Part model, mm, in its own coordinate system. A direction names the side the tool comes from. Give positions to 0.01 mm unless a question says otherwise; leave off trailing zeros. Order: outer loops, then holes, each group sorted by start corner. A loop starts at its lowest first (then second) coordinate and runs counter-clockwise, first axis right, second up. Notation, with made-up numbers: (24, 21.5) -> (35, 21.5) arc R31 ccw to (35, 60.5) -> close; hole circle Ø4 at (70, 53). An arc over 180 degrees is marked (long way). Write item = value, one per line. Start each with the question number.
(1) Probe line 1 along X through (y, z) = (55.5, -45.5); line 2 along X through (y, z) = (41, -36.5); line 3 along X through (y, z) = (91, 16). List the from-to ranges inside material, lowest first. Write a range as from..to.
(2) Flat gauge pins, fed straight in: pin 1 (1 mm diameter, centred on x = 61.5, z = -11.5, fed in from +Y); pin 2 (3 mm diameter, centred on x = 56, z = -33.5, fed in from +Y); pin 3 (1.5 mm diameter, centred on x = 82, y = 50.5, fed in from -Z). Where does each tip first touch, or does it go through?
(3) Saw through at A-A, the plane z = -68. List the corners of the cut face in (x, y), then the cut area to 3 significant figures.
(4) Which spindle directions (+Z, -Z, +X, -X, +Y, -Y) get a long thin tool onto all of the face, cutting with end or side? Do faces 5 (the cylindrical face through (56.1, 69.3, -48.9)), 6 (the flat face through (-9, 101.6, -35)). Say none if no direction does.
(5) Two-plate mould, pull along Y, no slides. Class faces 1 (the flat face through (33.566, 63.554, -20.049)), 2 (the flat face through (96.799, 21, -33)), 3 (the cylindrical face through (-8.706, 99.69, 24.452)), 4 (the cylindrical face through (34.07, 81.99, -33.91)): pulls with the +Y half, pulls with the -Y half, needs draft (parallel to the pull), parting line crosses it, or undercut.
from build123d import *

# Parameters (mm, degrees)
SKETCH1_W           = 120.65
SKETCH1_H           = 120.65
BOSS_EXTRUDE1_DEPTH = 101.6
CUT_EXTRUDE1_DEPTH  = 120.65
CUT_EXTRUDE2_DEPTH  = 31.75
CUT_EXTRUDE3_DEPTH  = 6.35
CUT_EXTRUDE3_TAPER  = 45
FILLET1_R           = 6.35
FILLET2_R           = 2.54


with BuildPart() as part:
    # Sketch1 → Boss-Extrude1 (new body)
    with BuildSketch(Plane(origin=(0, 0, 0), x_dir=(1, 0, 0), z_dir=(0, 1, 0))):
        with Locations((36.473705191, 34.061776503)):
            Rectangle(SKETCH1_W, SKETCH1_H)
    extrude(amount=BOSS_EXTRUDE1_DEPTH)

    # Sketch3 → Cut-Extrude1 (cut)
    with BuildSketch(Plane.XY.offset(26.263223497)):
        Polygon((96.798705191, 101.6), (1.548705191, 101.6), (96.798705191, 46.60738686), align=None)
    extrude(amount=-CUT_EXTRUDE1_DEPTH, mode=Mode.SUBTRACT)

    # Sketch4 → Cut-Extrude2 (cut)
    with BuildSketch(Plane(origin=(44.38126681, 76.870609019, 0), x_dir=(0.866025404, -0.5, 0), z_dir=(0.5, 0.866025404, 0))):
        Polygon((5.533831179, 52.832588454), (-10.722168821, 43.447182479), (-10.722168821, 24.676370527), (5.533831179, 15.290964551), (21.789831179, 24.676370527), (21.789831179, 43.447182479), align=None)
    extrude(amount=-CUT_EXTRUDE2_DEPTH, mode=Mode.SUBTRACT)

    # Sketch5 → Cut-Extrude3 (cut)
    with BuildSketch(Plane(origin=(28.50626681, 49.374302449, 0), x_dir=(0.866025404, -0.5, 0), z_dir=(0.5, 0.866025404, 0))):
        Polygon((5.533831179, 15.290964551), (21.789831179, 24.676370527), (21.789831179, 43.447182479), (5.533831179, 52.832588454), (-10.722168821, 43.447182479), (-10.722168821, 24.676370527), align=None)
    extrude(amount=-CUT_EXTRUDE3_DEPTH, taper=CUT_EXTRUDE3_TAPER, mode=Mode.SUBTRACT)

    # Fillet1
    fillet1_edges = [part.edges().sort_by_distance(p)[0] for p in [
        (-11.151294809, 101.6, -94.386776503),
        (96.798705191, 23.30369343, -94.386776503),
        (96.798705191, 23.30369343, 26.263223497),
        (49.173705191, 74.10369343, -94.386776503),
        (96.798705191, 46.60738686, -34.061776503),
        (1.548705191, 101.6, -34.061776503),
        (49.173705191, 74.10369343, 26.263223497),
        (-23.851294809, 101.6, -34.061776503),
        (-11.151294809, 101.6, 26.263223497),
        (-23.851294809, 50.8, -94.386776503),
        (-23.851294809, 50.8, 26.263223497),
    ]]
    fillet(fillet1_edges, radius=FILLET1_R)

    # Fillet2
    fillet2_edges = [part.edges().sort_by_distance(p)[0] for p in [
        (56.212759673, 70.03969343, -48.139885467),
        (42.134650709, 78.16769343, -48.139885467),
        (35.095596227, 82.23169343, -34.061776503),
        (42.134650709, 78.16769343, -19.983667539),
        (56.212759673, 70.03969343, -19.983667539),
        (63.251814155, 65.97569343, -34.061776503),
    ]]
    fillet(fillet2_edges, radius=FILLET2_R)


solid = part.part
Results list:
q1.line_1 = -23.85..23.77, 53.1..81.4
q1.line_2 = -23.85..30.31, 48.83..96.8
q1.line_3 = -23.85..19.91
q2.pin_1 = 67.28
q2.pin_2 = 56.01
q2.pin_3 = -94.19
q3.outline = (-23.85, 0) -> (96.8, 0) -> (96.8, 42.94) arc R6.35 ccw to (93.62, 48.44) -> (3.02, 100.75) arc R6.35 ccw to (-0.15, 101.6) -> (-17.5, 101.6) arc R6.35 ccw to (-23.85, 95.25) -> close
q3.area = 9,630 mm^2
q4.face_5 = +Y
q4.face_6 = +Z, -Z, +X, -X, +Y
q5.face_1 = undercut
q5.face_2 = needs draft
q5.face_3 = pulls with the +Y half
q5.face_4 = undercut
